Source: CAD feature listing. Evaluate the final solid. Frame: model axes, mm. Give positions to 0.01 mm unless a question says otherwise; leave off trailing zeros. Write each loop counter-clockwise with the first axis right and the second up, starting at its lowest first coordinate (ties: lowest second). Pieces come first, ordered by that corner, then holes. Notation, with made-up numbers: M -31,68 L -23,68 A29 ccw -23,94 Z; hole C -6.75,85 d8. An arc over 180 degrees is marked long. Return JSON: item names as keys, results as strings.
```python
from build123d import *

# Parameters (mm, degrees)
F0_W     = 152.4
F0_H     = 38.1
F1_DEPTH = 152.4
F3_DEPTH = 304.801
F4_W     = 76.2
F4_H     = 38.1
F5_DEPTH = 304.801


with BuildPart() as f1:
    # F0 (on Front) → F1 (new body, symmetric)
    with BuildSketch(Plane.XZ):
        Rectangle(F0_W, F0_H)
    extrude(amount=F1_DEPTH, both=True)

    # F2 (on face) → F3 (cut, through all)
    with BuildSketch(Plane.XZ.offset(152.4)):
        Polygon((76.2, 19.05), (10.2088642316, 19.05), (76.2, -19.05), align=None)
    extrude(amount=-F3_DEPTH, mode=Mode.SUBTRACT)

    # F4 (on face) → F5 (cut, through all)
    with BuildSketch(Plane.XZ.offset(152.4)):
        with Locations((-38.1, 0)):
            Rectangle(F4_W, F4_H)
    extrude(amount=-F5_DEPTH, mode=Mode.SUBTRACT)


solid = f1.part
```
1) Cut plane B-B, the plane x = 65. Return the cut outline in (y, z).
Numbers:
{"outline": "M -152.4,-19.05 L 152.4,-19.05 L 152.4,-12.58 L -152.4,-12.58 Z"}
2) Line query: line 1 (X direction, y = 62.5, z = 7.5); line 2 (X direction, y = 34, z = 12); line 3 (Z direction, x = 36, y = 23). Output: solid intervals per line, ascending. Write a range as [from, to].
Numbers:
{"line 1": "x = [0, 30.21]", "line 2": "x = [0, 22.42]", "line 3": "z = [-19.05, 4.16]"}
3) Contact query for flat-ended pins moving along their axis: pin 1 Ø12 at (x, y) = (47, -17) entering from +Z; pin 2 Ø10 at (y, z) = (-85.5, -13.5) entering from +X. Output: stop coordinate, or through.
Numbers:
{"pin 1": "stops at z = 1.27", "pin 2": "stops at x = 75.25"}
4) Cut plane A-A, the plane y = -3.5. Return the cut outline in (x, z).
Numbers:
{"outline": "M 0,-19.05 L 76.2,-19.05 L 10.21,19.05 L 0,19.05 Z"}
